from build123d import *

# Parameters (mm, degrees)
SKETCH_3_R                  = 11
EXTRUDE_1_DEPTH             = 30
HOLE_WIZARD_M32_D           = 3.4
HOLE_WIZARD_M32_CBORE_D     = 6.5
HOLE_WIZARD_M32_CBORE_DEPTH = 3
SKETCH_15_R                 = 9.5
CUT_EXTRUDE_1_DEPTH         = 144.273479751


with BuildPart() as part:
    # Эскиз3 → Бобышка-Вытянуть1 (new body)
    with BuildSketch(Plane(origin=(0, 0, 0), x_dir=(1, 0, 0), z_dir=(0, 1, 0))):
        with BuildLine():
            Line((0, 0), (-60, 0))
            Line((-60, 0), (-60, 56.188060056))
            Line((-60, 56.188060056), (-50.5, 56.188060056))
            Line((-50.5, 56.188060056), (-50.5, 46.188060056))
            ThreePointArc((-50.5, 46.188060056), (-50, 36.21312287), (-49.5, 46.188060056))
            Line((-49.5, 46.188060056), (-49.5, 56.188060056))
            Line((-49.5, 56.188060056), (-40, 56.188060056))
            Line((-40, 56.188060056), (-40, 30))
            Line((-40, 30), (-21.15, 30))
            Line((-21.15, 30), (-21.15, 72.3))
            Line((-21.15, 72.3), (21.15, 72.3))
            Line((21.15, 72.3), (21.15, 30))
            Line((21.15, 30), (40, 30))
            Line((40, 30), (40, 56.188060056))
            Line((40, 56.188060056), (49.5, 56.188060056))
            Line((49.5, 56.188060056), (49.5, 46.188060056))
            ThreePointArc((49.5, 46.188060056), (50, 36.21312287), (50.5, 46.188060056))
            Line((50.5, 46.188060056), (50.5, 56.188060056))
            Line((50.5, 56.188060056), (60, 56.188060056))
            Line((60, 56.188060056), (60, 0))
            Line((60, 0), (0, 0))
        make_face()
        with Locations(Location((0, 51.15, 0), (0, 0, 270))):
            Circle(SKETCH_3_R, mode=Mode.SUBTRACT)
    extrude(amount=EXTRUDE_1_DEPTH)

    # Цековка для винта с внутренним шестигранником M32 (through all)
    with Locations(Plane(origin=(0, 30, 0), x_dir=(1, 0, 0), z_dir=(0, 1, 0))):
        with Locations((-15.5, 66.65), (15.5, 66.65), (15.5, 35.65), (-15.5, 35.65)):
            CounterBoreHole(HOLE_WIZARD_M32_D / 2, HOLE_WIZARD_M32_CBORE_D / 2, HOLE_WIZARD_M32_CBORE_DEPTH)

    # Эскиз15 → Вырез-Вытянуть1 (cut, through all)
    with BuildSketch(Plane.ZY.offset(60)):
        with Locations((-15, 15)):
            Circle(SKETCH_15_R)
    extrude(amount=-CUT_EXTRUDE_1_DEPTH, mode=Mode.SUBTRACT)


solid = part.part
Could you check a few things on this model? Use its own coordinates, in mm. A direction names the side the tool comes from. Give positions to 0.01 mm unless a question says otherwise; leave off trailing zeros. Order: outer loops, then holes, each group sorted by start corner. A loop starts at its lowest first (then second) coordinate and runs counter-clockwise, first axis right, second up. Notation, with made-up numbers: (-17.75, 84.5) -> (40.25, 84.5) arc R24 ccw to (40.25, 109.5) -> close; hole circle Ø1 at (57, 28). An arc over 180 degrees is marked (long way). Answer in a Markdown table with one row per item. Add a question column.
Item 1: For faces 4 (the cylindrical face through (15.077, 28.521, -69.872)), 5 (the flat face through (45, 15, -56.188)), 6 (the flat face through (49.5, 15, -51)), which set-ups out of +Z, -Z, +X, -X, +Y, -Y let a thin tool reach every point of the face, with its end or its side?
Item 2: Imagine slicing it at B-B (x = 15.5). List the corners of the cut face in (y, z) for me.
Item 3: We'd pull the mould along Z, two halves only. Please class faces 1 (the flat face through (-31, 15, -30)), 2 (the cylindrical face through (-15.923, 28.521, -69.872)), 3 (the flat face through (50.5, 15, -51)): pulls with the +Z half, pulls with the -Z half, needs draft (parallel to the pull), parting line crosses it, or undercut.
Item 4: Imagine slicing it at A-A (z = -66.65). List the corners of the cut face in (x, y) for me, and give its area (3 significant figures).
Item 5: Imagine slicing it at D-D (z = -51.15). List the corners of the cut face in (x, y) for me, and give its area (3 significant figures).
Item 6: Please list where these lines run through material, in increasing order: probe 1 along X at (y, z) = (28.5, -66.65); probe 2 along Z at (x, y) = (15.5, 27.7); probe 3 along Y at (x, z) = (23, -15).
Item 7: Imagine slicing it at C-C (y = 19.75). Count the separate pieces of the cut face and the enclosed holes in it, and give its area (3 significant figures).
Item 8: I'm going to push flat-ended pins straight in: P1, Ø7.5, axis at x = 43, y = 18.5, coming from the -Z side; P2, Ø6, axis at x = 50, z = -41.21, coming from the +Y side. Where does each tip first touch, or does it pass through?
Result:
| question | item | result |
|---|---|---|
| 1 | face 4 | +Y |
| 1 | face 5 | -Z, +X, +Y, -Y |
| 1 | face 6 | -Z, +Y, -Y |
| 2 | outline | (0, -72.3) -> (30, -72.3) -> (30, -69.9) -> (27, -69.9) -> (27, -68.35) -> (0, -68.35) -> close; (0, -64.95) -> (27, -64.95) -> (27, -63.4) -> (30, -63.4) -> (30, -38.9) -> (27, -38.9) -> (27, -37.35) -> (0, -37.35) -> close; (0, -33.95) -> (27, -33.95) -> (27, -32.4) -> (30, -32.4) -> (30, 0) -> (0, 0) -> close; hole circle Ø19 at (15, -15) |
| 3 | face 1 | pulls with the -Z half |
| 3 | face 2 | undercut |
| 3 | face 3 | needs draft |
| 4 | outline | (-21.15, 0) -> (-17.2, 0) -> (-17.2, 27) -> (-18.75, 27) -> (-18.75, 30) -> (-21.15, 30) -> close; (-13.8, 0) -> (13.8, 0) -> (13.8, 27) -> (12.25, 27) -> (12.25, 30) -> (-12.25, 30) -> (-12.25, 27) -> (-13.8, 27) -> close; (17.2, 0) -> (21.15, 0) -> (21.15, 30) -> (18.75, 30) -> (18.75, 27) -> (17.2, 27) -> close |
| 4 | area | 1,050 mm2 |
| 5 | outline | (-60, 0) -> (-50.5, 0) -> (-50.5, 30) -> (-60, 30) -> close; (-49.5, 0) -> (-40, 0) -> (-40, 30) -> (-49.5, 30) -> close; (-21.15, 0) -> (-11, 0) -> (-11, 30) -> (-21.15, 30) -> close; (11, 0) -> (21.15, 0) -> (21.15, 30) -> (11, 30) -> close; (40, 0) -> (49.5, 0) -> (49.5, 30) -> (40, 30) -> close; (50.5, 0) -> (60, 0) -> (60, 30) -> (50.5, 30) -> close |
| 5 | area | 1,750 mm2 |
| 6 | probe 1 | -21.15 to -18.75, -12.25 to 12.25, 18.75 to 21.15 |
| 6 | probe 2 | -72.3 to -69.9, -63.4 to -38.9, -32.4 to 0 |
| 6 | probe 3 | 0 to 5.5, 24.5 to 30 |
| 7 | separate pieces | 2 |
| 7 | enclosed holes | 5 |
| 7 | area | 3,870 mm2 |
| 8 | P1 | z = -56.19 |
| 8 | P2 | through |
